from build123d import *

# Parameters (mm, degrees)
BOSS_EXTRUDE1_DEPTH     = 37
CUT_EXTRUDE1_DEPTH      = 101.656930314
CUT_EXTRUDE1_DEPTH_BACK = 101.656930314
SKETCH6_R               = 7.5
CUT_EXTRUDE2_DEPTH      = 143.407678732
SKETCH7_R               = 7.5
CUT_EXTRUDE3_DEPTH      = 143.407678732
FILLET1_R               = 3


with BuildPart() as part:
    # Sketch3 → Boss-Extrude1 (new body)
    with BuildSketch(Plane(origin=(0, 0, 0), x_dir=(1, 0, 0), z_dir=(0, 1, 0))):
        Polygon((-59.997474683, 62.497474683), (-38.997474683, 62.497474683), (-38.997474683, 51.346717088), (51.346717088, -38.997474683), (62.497474683, -38.997474683), (62.497474683, -59.997474683), (36.497474683, -59.997474683), (36.497474683, -53.846717088), (-53.846717088, 36.497474683), (-59.997474683, 36.497474683), align=None)
    extrude(amount=BOSS_EXTRUDE1_DEPTH)

    # Sketch5 → Cut-Extrude1 (cut, two sides: drawn at the far end of the back side and taken through both)
    with BuildSketch(Plane(origin=(7.806349186, 0, -4.542893219), x_dir=(0.7071067811865459, 0, 0.7071067811865491), z_dir=(-0.7071067811865491, 0, 0.7071067811865459)).offset(-CUT_EXTRUDE1_DEPTH_BACK)):
        Polygon((61.575378798, 37), (12.192388155, 37), (12.192388155, 23.5), (84.309397513, 23.5), (84.309397513, 37), (69.460155108, 37), align=None)
        Polygon((-9.807611845, 0), (-66.190602487, 0), (-74.075378798, 0), (-88.924621202, 0), (-88.924621202, 13.5), (-9.807611845, 13.5), align=None)
    extrude(amount=CUT_EXTRUDE1_DEPTH + CUT_EXTRUDE1_DEPTH_BACK, mode=Mode.SUBTRACT)

    # Sketch6 → Cut-Extrude2 (cut, through all)
    with BuildSketch(Plane(origin=(62.497474683, 0, 0), x_dir=(0, 0, -1), z_dir=(1, 0, 0))):
        with Locations((-49.497474683, 11.75)):
            Circle(SKETCH6_R)
    extrude(amount=-CUT_EXTRUDE2_DEPTH, mode=Mode.SUBTRACT)

    # Sketch7 → Cut-Extrude3 (cut, through all)
    with BuildSketch(Plane(origin=(0, 0, -62.497474683), x_dir=(-1, 0, 0), z_dir=(0, 0, -1))):
        with Locations((49.497474683, 25.25)):
            Circle(SKETCH7_R)
    extrude(amount=-CUT_EXTRUDE3_DEPTH, mode=Mode.SUBTRACT)

    # Fillet1
    fillet1_edges = [part.edges().sort_by_distance(p)[0] for p in [
        (56.922095886, 0, 38.997474683),
        (56.922095886, 23.5, 38.997474683),
        (-38.997474683, 25.25, -51.346717088),
        (26.109018716, 0, 13.759776311),
        (51.346717088, 11.75, 38.997474683),
        (33.887193309, 23.5, 21.537950904),
        (62.497474683, 0, 49.497474683),
        (62.497474683, 11.75, 59.997474683),
        (62.497474683, 23.5, 49.497474683),
        (62.497474683, 11.75, 38.997474683),
        (-6.553300859, 0, -4.053300859),
        (-33.912319575, 13.5, -16.56307717),
        (-19.06307717, 13.5, -31.412319575),
        (-38.997474683, 13.5, -56.922095886),
        (-56.922095886, 13.5, -36.497474683),
        (-59.997474683, 25.25, -36.497474683),
        (-59.997474683, 13.5, -49.497474683),
        (-59.997474683, 25.25, -62.497474683),
        (-49.497474683, 13.5, -62.497474683),
        (-38.997474683, 25.25, -62.497474683),
        (-26.134144982, 37, -8.784902577),
        (-56.922095886, 37, -36.497474683),
        (-59.997474683, 37, -49.497474683),
        (-49.497474683, 37, -62.497474683),
        (-38.997474683, 37, -56.922095886),
        (-11.284902577, 37, -23.634144982),
        (9.003048327, 37, 11.503048327),
        (19.037950904, 23.5, 36.387193309),
        (11.259776311, 0, 28.609018716),
        (49.497474683, 0, 59.997474683),
        (49.497474683, 23.5, 59.997474683),
        (36.497474683, 11.75, 59.997474683),
        (36.497474683, 0, 56.922095886),
        (-53.846717088, 16.319918557, -36.497474683),
        (-53.846717088, 34.180081443, -36.497474683),
        (36.497474683, 20.680081443, 53.846717088),
        (36.497474683, 2.819918557, 53.846717088),
        (36.497474683, 23.5, 56.922095886),
    ]]
    fillet(fillet1_edges, radius=FILLET1_R - 0.0001)  # a hair under: the kernel refuses the full size


solid = part.part
Input: part model. Units: mm. Frame: model coordinates. A direction names the side the tool comes from. Round coordinates to 2 decimals unless told otherwise and drop trailing zeros. Answer as a JSON object with one key per item and string values. Group by question number.
1) Pin query (flat end, axial travel): pin 1 (15 mm diameter, centred on x = 26, z = 20.5, fed in from +Y); pin 2 (8 mm diameter, centred on x = -37.5, y = 22, fed in from +Z); pin 3 (1 mm diameter, centred on y = 9, z = 56, fed in from -X). Return the tip coordinate at first contact, or that it passes through.
2) Ray query, L1, parallel to X at y = 25.25, z = -54; L2, parallel to X at y = 25.25, z = -48; L3, parallel to Z at x = 52, y = 11. Return the intervals inside material, ascending.
3) Reachability of faces 1 (the cylindrical face through (-39.9, 14.355, -55.995)), 2 (the cylindrical face through (37.4, 0.855, 56.03)), 3 (the flat face through (-38.997, 25, -56)) from +Z, -Z, +X, -X, +Y, -Y: full face, straight path, thin tool, end or side. Return the list, or none.
Reply:
{
 "1": {"pin 1": "stops at y = 23.5", "pin 2": "stops at z = -16.15", "pin 3": "stops at x = 36.5"},
 "2": {"L1": "x = -60 to -57, -42 to -39", "L2": "x = -60 to -57, -42 to -35.65", "L3": "z = 38.94 to 42.04, 56.96 to 60"},
 "3": {"face 1": "-Z, +X, -Y", "face 2": "+Z, -X, -Y", "face 3": "-Z, +X, +Y, -Y"}
}
